Answer from the drawing. Dimensions are ordinates in mm from the lowest x, y and z of the part. Give positions to 0.01 mm unless a question says otherwise; leave off trailing zeros. Order: outer loops, then holes, each group sorted by start corner. A loop starts at its lowest first (then second) coordinate and runs counter-clockwise, first axis right, second up. Notation, with made-up numbers: (34.25, -12) - (53.25, -12) arc R30 cw to (53.25, 14) - close; hole circle Ø3 at (-9.75, 28). An arc over 180 degrees is marked (long way). Use a Markdown table: item, result. Add a question column.
1) Straight lines are drawn through the part: line 1 (X direction, y = 0.35, z = 34); line 2 (X direction, y = 0.5, z = 44); line 3 (Z direction, x = 3.5, y = 1.35). For each, find the intervals that lie inside material, in ascending order.
2) Find section A-A, the plane y = 1. Determine the outline of the cut face in (x, z).
3) Flat-ended cylindrical pins translate along their axes: pin 1 (0.5 mm diameter, centred on x = 25, y = 0.5, fed in from +Z); pin 2 (0.5 mm diameter, centred on x = 24, y = 0.5, fed in from -Z). Find the tip coordinate at first contact, or state that the pin passes through.
4) Find section C-C, the plane x = 54. Determine the outline of the cut face in (y, z).
5) Find section D-D, the plane z = 13. Determine the outline of the cut face in (x, y).
6) Find section B-B, the plane z = 39. Determine the outline of the cut face in (x, y).
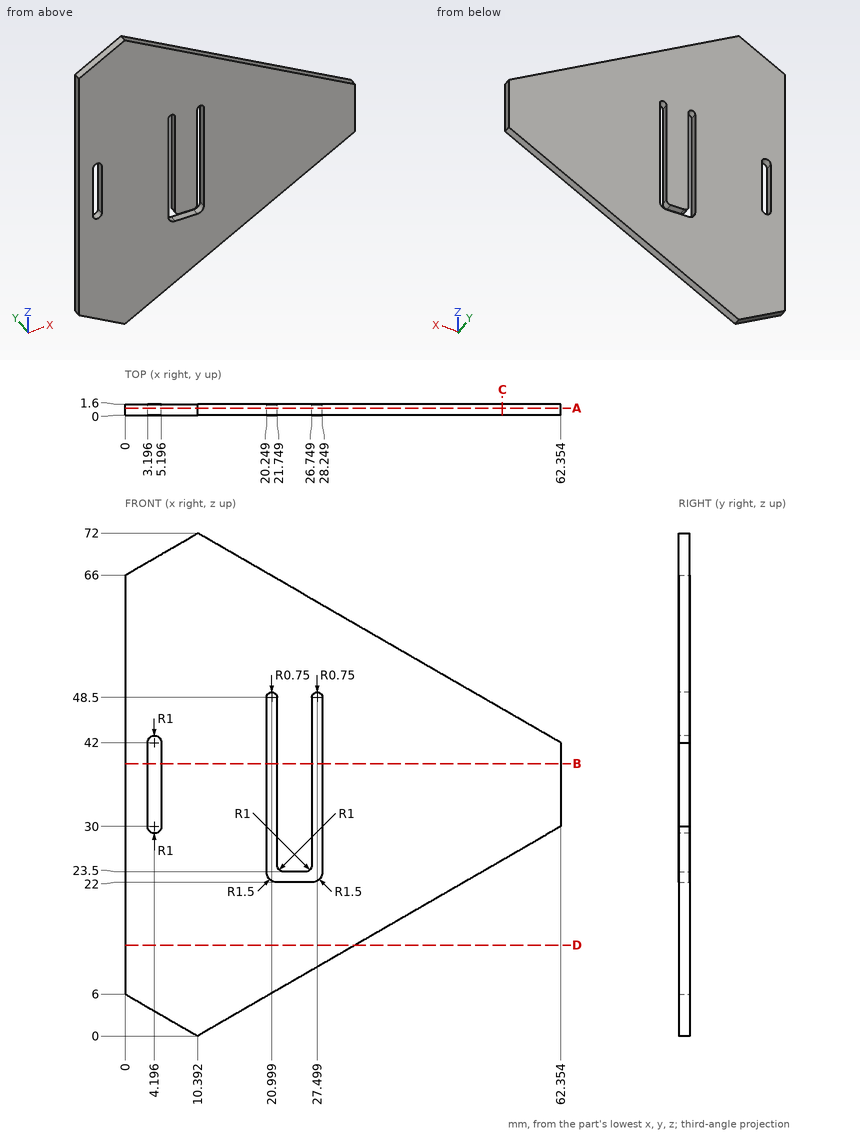
The answers:
| question | item | result |
|---|---|---|
| 1 | line 1 | 0 to 3.2, 5.2 to 20.25, 21.75 to 26.75, 28.25 to 62.35 |
| 1 | line 2 | 0 to 20.25, 21.75 to 26.75, 28.25 to 58.89 |
| 1 | line 3 | 3.98 to 29.28, 42.72 to 68.02 |
| 2 | outline | (0, 6) - (10.39, 0) - (62.35, 30) - (62.35, 42) - (10.39, 72) - (0, 66) - close; hole (3.2, 30) arc R1 ccw to (5.2, 30) - (5.2, 42) arc R1 ccw to (3.2, 42) - close; hole (20.25, 23.5) arc R1.5 ccw to (21.75, 22) - (26.75, 22) arc R1.5 ccw to (28.25, 23.5) - (28.25, 48.5) arc R0.75 ccw to (26.75, 48.5) - (26.75, 24.5) arc R1 cw to (25.75, 23.5) - (22.75, 23.5) arc R1 cw to (21.75, 24.5) - (21.75, 48.5) arc R0.75 ccw to (20.25, 48.5) - close |
| 3 | pin 1 | z = 63.71 |
| 3 | pin 2 | z = 7.71 |
| 4 | outline | (0, 25.18) - (1.6, 25.18) - (1.6, 46.82) - (0, 46.82) - close |
| 5 | outline | (0, 0) - (32.91, 0) - (32.91, 1.6) - (0, 1.6) - close |
| 6 | outline | (0, 0) - (3.2, 0) - (3.2, 1.6) - (0, 1.6) - close; (5.2, 0) - (20.25, 0) - (20.25, 1.6) - (5.2, 1.6) - close; (21.75, 0) - (26.75, 0) - (26.75, 1.6) - (21.75, 1.6) - close; (28.25, 0) - (62.35, 0) - (62.35, 1.6) - (28.25, 1.6) - close |
